The listing builds one solid part. Answer for the finished solid, in the listing's coordinates (mm). Coordinates: 2 decimals unless noted, no trailing zeros. Write each loop counter-clockwise with the first axis right and the second up, starting at its lowest first coordinate (ties: lowest second). Pieces come first, ordered by that corner, then holes.
from build123d import *

# Parameters (mm, degrees)
BOSS_EXTRUDE1_DEPTH = 235
SKETCH3_R           = 1.75
CUT_EXTRUDE2_DEPTH  = 237.535409611
CHAMFER1_SIZE       = 3
SKETCH4_R           = 1.75
CUT_EXTRUDE3_DEPTH  = 237.535409611


with BuildPart() as part:
    # Sketch1 → Boss-Extrude1 (new, symmetric)
    with BuildSketch(Plane.XY):
        Polygon((0, 0), (20, 0), (20, 2), (2, 2), (2, 20), (0, 20), align=None)
    extrude(amount=BOSS_EXTRUDE1_DEPTH, both=True)

    # Cut-Extrude1 cone 1 section (through the dimple's axis) → Cut-Extrude1 (revolve, cut)
    with BuildSketch(Plane(origin=(11, 2, -220), x_dir=(0, 0, 1), z_dir=(1, 0, 0))):
        Polygon((0, 0), (3.5, 0), (0, 3.5), align=None)
    revolve(axis=Axis((11, 2, -220), (0, -1, 0)), mode=Mode.SUBTRACT)

    # Cut-Extrude1 cone 2 section (through the dimple's axis) → Cut-Extrude1 cone 2 (revolve, cut)
    with BuildSketch(Plane(origin=(11, 2, 220), x_dir=(0, 0, 1), z_dir=(1, 0, 0))):
        Polygon((0, 0), (3.5, 0), (0, 3.5), align=None)
    revolve(axis=Axis((11, 2, 220), (0, -1, 0)), mode=Mode.SUBTRACT)

    # Sketch3 → Cut-Extrude2 (cut, through all)
    with BuildSketch(Plane(origin=(0, 2, 0), x_dir=(1, 0, 0), z_dir=(0, 1, 0))):
        with Locations(Location((11, -220, 0), (0, 0, 180))):
            Circle(SKETCH3_R)
        with Locations(Location((11, 220, 0), (0, 0, 180))):
            Circle(SKETCH3_R)
    extrude(amount=-CUT_EXTRUDE2_DEPTH, mode=Mode.SUBTRACT)

    # Chamfer1
    chamfer1_edges = [part.edges().sort_by_distance(p)[0] for p in [
        (20, 1, 235),
        (1, 20, 235),
        (1, 20, -235),
        (20, 1, -235),
    ]]
    chamfer(chamfer1_edges, length=CHAMFER1_SIZE)

    # Sketch4 → Cut-Extrude3 (cut, through all)
    with BuildSketch(Plane(origin=(0, 2, 0), x_dir=(1, 0, 0), z_dir=(0, 1, 0))):
        with Locations(Location((12, 144, 0), (0, 0, 180))):
            Circle(SKETCH4_R)
        with Locations(Location((12, -114, 0), (0, 0, 180))):
            Circle(SKETCH4_R)
    extrude(amount=-CUT_EXTRUDE3_DEPTH, mode=Mode.SUBTRACT)


solid = part.part
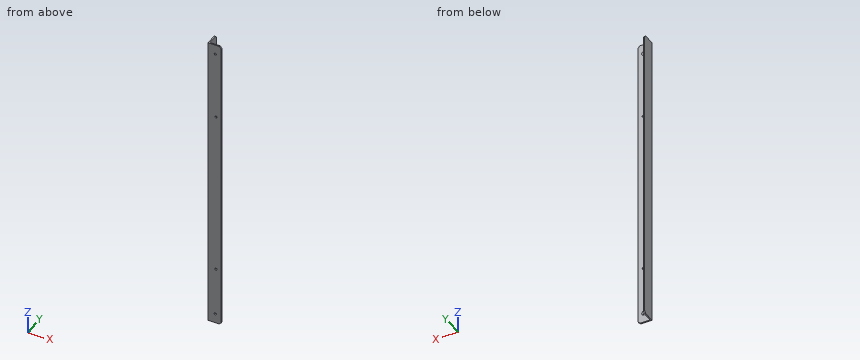
Q1. Find the intervals of material crossed by probe 1 along X at (y, z) = (0.7, -144); probe 2 along Z at (x, y) = (12, 1.2); probe 3 along Z at (x, y) = (11, 0.25), in increasing order.
Answers below:
probe 1: x = 0 to 10.25, 13.75 to 20
probe 2: z = -235 to -222.51, -217.49 to -145.75, -142.25 to 112.25, 115.75 to 217.49, 222.51 to 235
probe 3: z = -235 to -221.75, -218.25 to -145.44, -142.56 to 112.56, 115.44 to 218.25, 221.75 to 235
Q2. The part is cut by section B-B, the plane y = 8.25. Write down the section's boundary in (x, z).
Answers below:
outline: (0, -235) - (2, -235) - (2, 235) - (0, 235) - close
Q3. Given pin 1 (8 mm diameter, centred on x = 6, y = 4, fed in from -Z); pin 2 (1 mm diameter, centred on y = 13.5, z = 64, fed in from +X); pin 3 (2 mm diameter, centred on x = 12, z = 114, fed in from +Y); pin 4 (9 mm diameter, centred on x = 11, z = 76, fed in from +Y), each flat-ended and moving along its own axis, determine where each tip first touches the part or whether it passes through.
Answers below:
pin 1: stops at z = -235
pin 2: stops at x = 2
pin 3: passes through
pin 4: stops at y = 2
Q4. The part is cut by section A-A, the plane z = -106. Write down the section's boundary in (x, y), then the cut area to 3 significant figures.
Answers below:
outline: (0, 0) - (20, 0) - (20, 2) - (2, 2) - (2, 20) - (0, 20) - close
area: 76.0 mm2
